Geometry check sheet. Reference: drawing and pictorial views, mm from the part's lowest x, y, z. Coordinates: 2 decimals unless noted, no trailing zeros. Write each loop counter-clockwise with the first axis right and the second up, starting at its lowest first coordinate (ties: lowest second). Pieces come first, ordered by that corner, then holes.
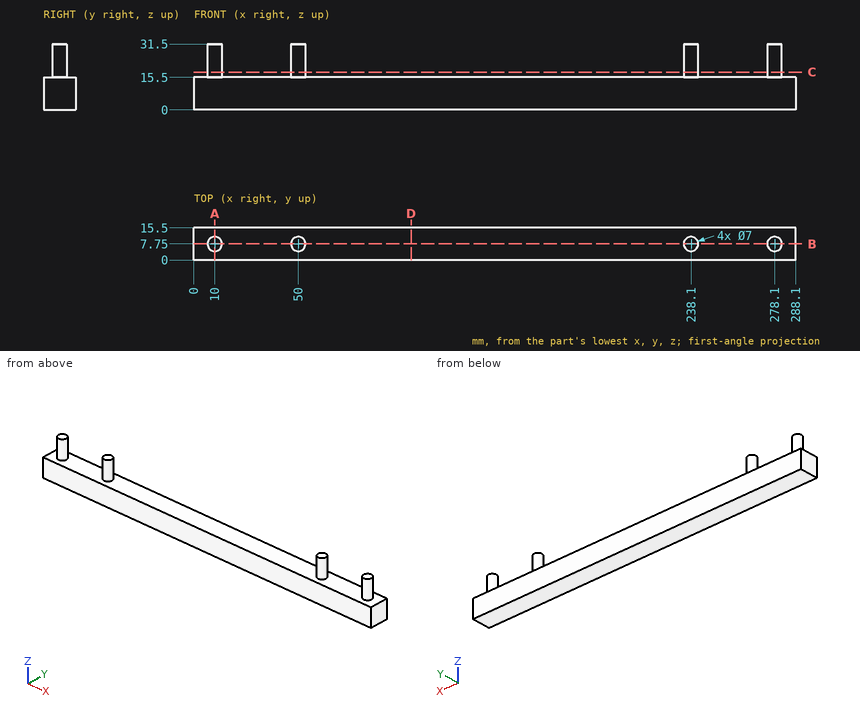
1. Sectioned sample at A-A, the plane x = 10. Record the boundary of the cut face in (y, z), and give its area (3 significant figures).
2. Material ranges on L1, parallel to X at y = 8, z = 16; L2, parallel to Z at x = 110.5, y = 12.25, recorded low to high.
3. Sectioned sample at D-D, the plane x = 104. Record the boundary of the cut face in (y, z), and give its area (3 significant figures).
4. Sectioned sample at B-B, the plane y = 7.75. Record the boundary of the cut face in (x, z).
5. Sectioned sample at C-C, the plane z = 18. Record the boundary of the cut face in (x, y), and give its area (3 significant figures).
6. Gauge pin test, flat ends, axial feed: P1, Ø2, axis at y = 6, z = 19.5, coming from the -X side; P2, Ø8, axis at x = 184, y = 9, coming from the +Z side; P3, Ø12, axis at x = 30.5, z = 23.5, coming from the +Y side. Record the tip position at first contact, or that the pin passes through.
Outcome:
1. outline: (0, 0) - (15.5, 0) - (15.5, 15.5) - (11.25, 15.5) - (11.25, 31.5) - (4.25, 31.5) - (4.25, 15.5) - (0, 15.5) - close
1. area: 352 mm2
2. L1: x = 6.51 to 13.49, 46.51 to 53.49, 234.61 to 241.59, 274.61 to 281.59
2. L2: z = 0 to 15.5
3. outline: (0, 0) - (15.5, 0) - (15.5, 15.5) - (0, 15.5) - close
3. area: 240 mm2
4. outline: (0, 0) - (288.1, 0) - (288.1, 15.5) - (281.6, 15.5) - (281.6, 31.5) - (274.6, 31.5) - (274.6, 15.5) - (241.6, 15.5) - (241.6, 31.5) - (234.6, 31.5) - (234.6, 15.5) - (53.5, 15.5) - (53.5, 31.5) - (46.5, 31.5) - (46.5, 15.5) - (13.5, 15.5) - (13.5, 31.5) - (6.5, 31.5) - (6.5, 15.5) - (0, 15.5) - close
5. outline: circle Ø7 at (10, 7.75); circle Ø7 at (50, 7.75); circle Ø7 at (238.1, 7.75); circle Ø7 at (278.1, 7.75)
5. area: 154 mm2
6. P1: stops at x = 6.58
6. P2: stops at z = 15.5
6. P3: passes through
